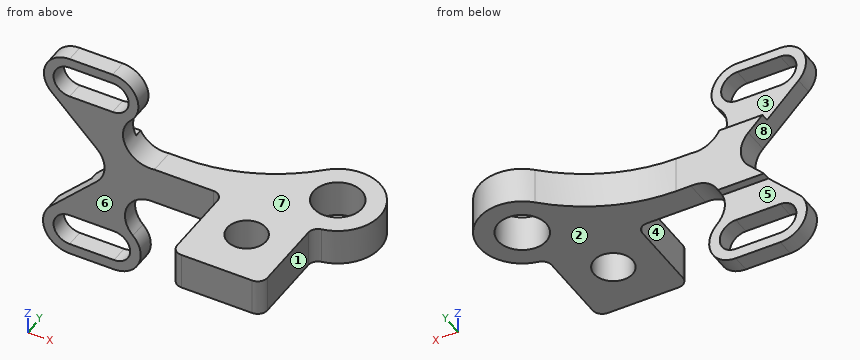
```python
from build123d import *

# Parameters (mm, degrees)
BOSS_EXTRUDE1_DEPTH = 16
BOSS_EXTRUDE2_START = -22.627417
SKETCH2_R           = 12
SKETCH2_R_2         = 15
BOSS_EXTRUDE2_DEPTH = 22.627417
FILLET1_R           = 6
SKETCH6_W           = 59.235505044
SKETCH6_H           = 5
CUT_EXTRUDE3_DEPTH  = 46.82239
SKETCH9_W           = 60.661911653
SKETCH9_H           = 5
CUT_EXTRUDE4_DEPTH  = 47.281077


with BuildPart() as part:
    # Sketch1 → Boss-Extrude1 (new body)
    with BuildSketch(Plane(origin=(0, 0, 0), x_dir=(1, 0, 0), z_dir=(0, 1, 0))):
        with BuildLine():
            Line((-46.084327379, 32.649418524), (-18.51965158, 32.649418524))
            ThreePointArc((-18.51965158, 32.649418524), (-3.230722186, 22.433682506), (-6.818011624, 4.399160642))
            ThreePointArc((-6.818011624, 4.399160642), (-10.165791884, -14.631658747), (6.580056768, -24.273042062))
            Line((6.580056768, -24.273042062), (89.580056768, -24.273042062))
            Line((89.580056768, -24.273042062), (89.580056768, -46.90045906))
            Line((89.580056768, -46.90045906), (6.580056768, -46.90045906))
            ThreePointArc((6.580056768, -46.90045906), (-11.103107382, -55.676049041), (-8.083731763, -75.184730307))
            ThreePointArc((-8.083731763, -75.184730307), (-4.615367742, -92.621373724), (-19.397440262, -102.498438806))
            Line((-19.397440262, -102.498438806), (-46.084327379, -102.498438806))
            ThreePointArc((-46.084327379, -102.498438806), (-60.866399899, -92.621373724), (-57.398035878, -75.184730307))
            Line((-57.398035878, -75.184730307), (-29.113764631, -46.90045906))
            ThreePointArc((-29.113764631, -46.90045906), (-24.42747313, -35.586750561), (-29.113764631, -24.273042062))
            Line((-29.113764631, -24.273042062), (-57.785967334, 4.399160642))
            ThreePointArc((-57.785967334, 4.399160642), (-61.373256773, 22.433682506), (-46.084327379, 32.649418524))
        make_face()
        with BuildLine():
            Line((-46.084327379, 26.100800597), (-18.51965158, 26.100800597))
            ThreePointArc((-18.51965158, 26.100800597), (-8.51965158, 16.100800597), (-18.51965158, 6.100800597))
            Line((-18.51965158, 6.100800597), (-46.084327379, 6.100800597))
            ThreePointArc((-46.084327379, 6.100800597), (-56.084327379, 16.100800597), (-46.084327379, 26.100800597))
        make_face(mode=Mode.SUBTRACT)
        with BuildLine():
            Line((-46.084327379, -76.498438806), (-19.397440262, -76.498438806))
            ThreePointArc((-19.397440262, -76.498438806), (-9.397440262, -86.498438806), (-19.397440262, -96.498438806))
            Line((-19.397440262, -96.498438806), (-46.084327379, -96.498438806))
            ThreePointArc((-46.084327379, -96.498438806), (-56.084327379, -86.498438806), (-46.084327379, -76.498438806))
        make_face(mode=Mode.SUBTRACT)
    extrude(amount=BOSS_EXTRUDE1_DEPTH)

    # Sketch2 → Boss-Extrude2 (add)
    with BuildSketch(Plane.XY.offset(46.90045906).offset(BOSS_EXTRUDE2_START)):
        with BuildLine():
            Line((105.185672621, -56), (105.185672621, 0))
            ThreePointArc((105.185672621, 0), (129.714674209, 36.710245129), (86.41198758, 45.323685041))
            ThreePointArc((86.41198758, 45.323685041), (53.931590324, 23.620977443), (15.618349457, 16))
            Line((15.618349457, 16), (89.580056768, 16))
            Line((89.580056768, 16), (89.580056768, 0))
            Line((89.580056768, 0), (49.185672621, 0))
            Line((49.185672621, 0), (49.185672621, -56))
            Line((49.185672621, -56), (105.185672621, -56))
        make_face()
        with Locations((77.185672621, -23.45)):
            Circle(SKETCH2_R, mode=Mode.SUBTRACT)
        with Locations((105.185672621, 26.55)):
            Circle(SKETCH2_R_2, mode=Mode.SUBTRACT)
    extrude(amount=BOSS_EXTRUDE2_DEPTH)

    # Fillet1
    fillet1_edges = [part.edges().sort_by_distance(p)[0] for p in [
        (105.185672621, 0, 35.58675056),
        (105.185672621, -56, 35.58675056),
        (49.185672621, -56, 35.58675056),
        (49.185672621, 0, 35.58675056),
    ]]
    fillet(fillet1_edges, radius=FILLET1_R)

    # Sketch6 → Cut-Extrude3 (cut)
    with BuildSketch(Plane.XY.offset(102.498438806)):
        with Locations((-33.015192784, 13.5)):
            Rectangle(SKETCH6_W, SKETCH6_H)
    extrude(amount=-CUT_EXTRUDE3_DEPTH, mode=Mode.SUBTRACT)

    # Sketch9 → Cut-Extrude4 (cut)
    with BuildSketch(Plane(origin=(0, 0, -32.649418524), x_dir=(-1, 0, 0), z_dir=(0, 0, -1))):
        with Locations((32.30198948, 13.5)):
            Rectangle(SKETCH9_W, SKETCH9_H)
    extrude(amount=-CUT_EXTRUDE4_DEPTH, mode=Mode.SUBTRACT)


solid = part.part
```
Build history of the part. All positions in model axes, mm. Face numbers are marked on the shaded views. A direction names the side the tool comes from. Coordinates: 2 decimals unless noted, no trailing zeros. Order: outer loops, then holes, each group sorted by start corner. A loop starts at its lowest first (then second) coordinate and runs counter-clockwise, first axis right, second up.
Item 1: Tool access for the marked faces 1, 2, 3, 4 and 5: list every direction of +Z, -Z, +X, -X, +Y, -Y with a clear straight run to the whole face (end or side of a thin tool).
Filled in:
face 1: +Z, -Z, +X, -Y
face 2: -Z, +X, +Y, -Y
face 3: +Z, +X, -X, +Y
face 4: +Z, -Z, -X, -Y
face 5: -Z, +X, -X, +Y
Item 2: Drop flat-ended pins along their axis: pin 1 Ø1 at (x, z) = (48, 30.5) entering from -Y; pin 2 Ø12 at (x, y) = (17, -5.5) entering from +Z; pin 3 Ø4 at (x, y) = (-21.5, 13.5) entering from -Z. Give the stop position or say it passes through.
Filled in:
pin 1: stops at y = -3.21
pin 2: stops at z = 46.9
pin 3: stops at z = 14.63
Item 3: Saw through at A-A on y = -23.45. List the corners of the cut face in (x, z), then the cut area to 3 significant figures.
Filled in:
outline: (49.19, 24.27) - (65.19, 24.27) - (65.19, 46.9) - (49.19, 46.9) - close; (89.19, 24.27) - (105.19, 24.27) - (105.19, 46.9) - (89.19, 46.9) - close
area: 724 mm2
Item 4: Mould opens along Z. For the marked faces 6, 7 and 8 say: released by +Z, released by -Z, zero draft, split by the parting line, or undercut.
Filled in:
face 6: zero draft
face 7: released by +Z
face 8: undercut
Item 5: Drill centre lines: L1, parallel to X at y = 26, z = 40; L2, parallel to Y at x = 101, z = 36; L3, parallel to Y at x = 1, z = 36. Where is each one in solid material? Low to high.
Filled in:
L1: x = 59.23 to 90.2, 120.18 to 131.73
L2: y = -55.72 to 12.15, 40.95 to 52.77
L3: y = 0 to 16
Item 6: Saw through at C-C on y = -42. List the corners of the cut face in (x, z), then the cut area to 3 significant figures.
Filled in:
outline: (49.19, 24.27) - (105.19, 24.27) - (105.19, 46.9) - (49.19, 46.9) - close
area: 1,270 mm2
Item 7: Saw through at D-D on x = 63. List the corners of the cut face in (y, z), then the cut area to 3 significant figures.
Filled in:
outline: (-56, 24.27) - (27.92, 24.27) - (27.92, 46.9) - (-56, 46.9) - close
area: 1,900 mm2
Item 8: Saw through at B-B on z = -13. List the corners of the cut face in (x, y).
Filled in:
outline: (-62.34, 0) - (-55.59, 0) - (-55.59, 11) - (-62.34, 11) - close; (-9.01, 0) - (-2.26, 0) - (-2.26, 11) - (-9.01, 11) - close
